Source: three-view drawing plus pictorial views. Frame: mm from the lowest corner of the part. Give positions to 0.01 mm unless a question says otherwise; leave off trailing zeros. Write each loop counter-clockwise with the first axis right and the second up, starting at its lowest first coordinate (ties: lowest second). Pieces come first, ordered by that corner, then holes.
Q1. Draft query along Z for the marked faces 1, 2 and 3. Return one class per face: pulls with the +Z half, pulls with the -Z half, needs draft (parallel to the pull), parting line crosses it, or undercut.
Q2. Pin query (flat end, axial travel): pin 1 (3.5 mm diameter, centred on x = 35.2, z = 51.45, fed in from -Y). Return the tip coordinate at first contact, or that it passes through.
Q3. Cut plane B-B on y = 0.85. Return the cut outline in (x, z), plus the area to 3 significant figures.
Q4. Cut plane D-D on z = 27.5. Return the cut outline in (x, y).
Q5. Cut plane A-A on x = 3.3. Return the cut outline in (y, z).
Q6. Line query: L1, parallel to Z at x = 3.3, y = 4.35; L2, parallel to Z at x = 35.2, y = 1.9; L3, parallel to X at y = 0.75, z = 52. Output: solid intervals per line, ascending.
Q7. Cut plane C-C on z = 3.55. Return the cut outline in (x, y).
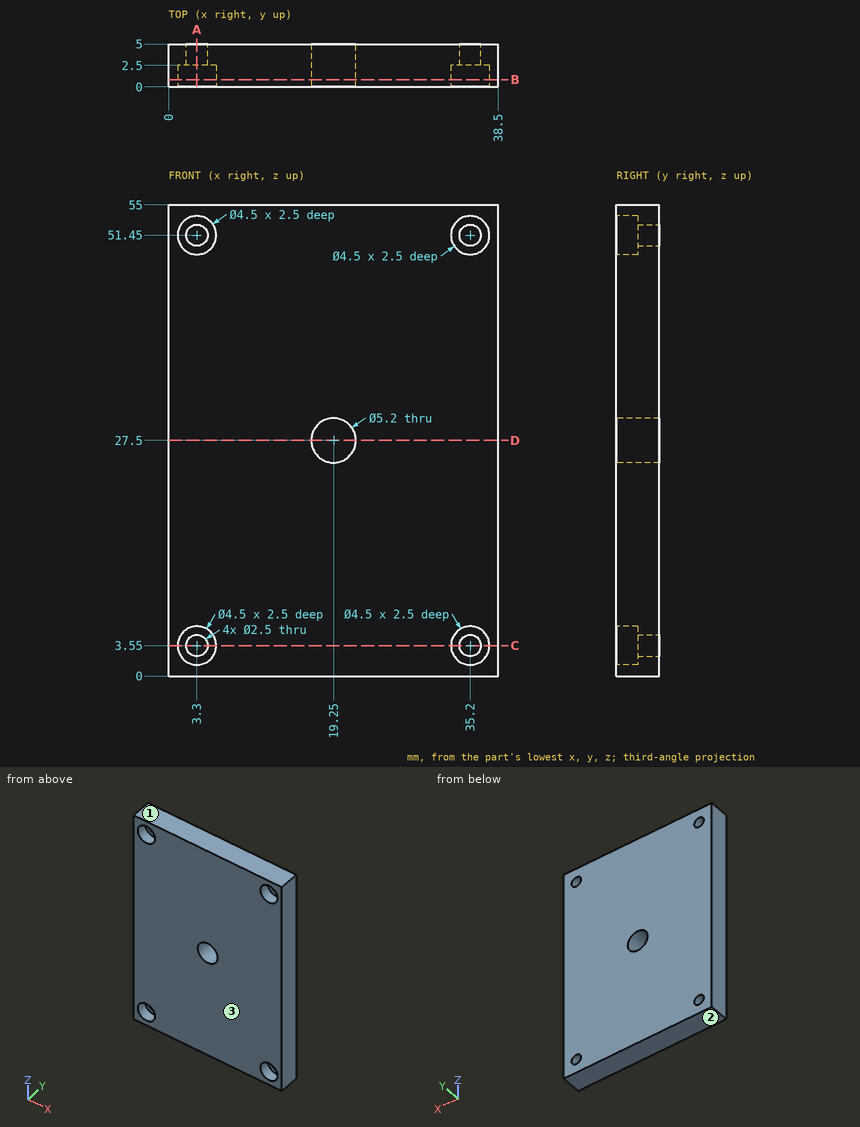
Data:
1. face 1: pulls with the +Z half
1. face 2: pulls with the -Z half
1. face 3: needs draft
2. pin 1: stops at y = 2.5
3. outline: (0, 0) - (38.5, 0) - (38.5, 55) - (0, 55) - close; hole circle Ø4.5 at (3.3, 3.55); hole circle Ø4.5 at (3.3, 51.45); hole circle Ø5.2 at (19.25, 27.5); hole circle Ø4.5 at (35.2, 3.55); hole circle Ø4.5 at (35.2, 51.45)
3. area: 2,030 mm2
4. outline: (0, 0) - (16.65, 0) - (16.65, 5) - (0, 5) - close; (21.85, 0) - (38.5, 0) - (38.5, 5) - (21.85, 5) - close
5. outline: (0, 0) - (5, 0) - (5, 2.3) - (2.5, 2.3) - (2.5, 1.3) - (0, 1.3) - close; (0, 5.8) - (2.5, 5.8) - (2.5, 4.8) - (5, 4.8) - (5, 50.2) - (2.5, 50.2) - (2.5, 49.2) - (0, 49.2) - close; (0, 53.7) - (2.5, 53.7) - (2.5, 52.7) - (5, 52.7) - (5, 55) - (0, 55) - close
6. L1: z = 0 to 2.3, 4.8 to 50.2, 52.7 to 55
6. L2: z = 0 to 1.3, 5.8 to 49.2, 53.7 to 55
6. L3: x = 0 to 1.12, 5.48 to 33.02, 37.38 to 38.5
7. outline: (0, 0) - (1.05, 0) - (1.05, 2.5) - (2.05, 2.5) - (2.05, 5) - (0, 5) - close; (4.55, 2.5) - (5.55, 2.5) - (5.55, 0) - (32.95, 0) - (32.95, 2.5) - (33.95, 2.5) - (33.95, 5) - (4.55, 5) - close; (36.45, 2.5) - (37.45, 2.5) - (37.45, 0) - (38.5, 0) - (38.5, 5) - (36.45, 5) - close
